Model file for the job. Use its own axes, mm. Face numbers are marked on the shaded views. Give positions to 0.01 mm unless a question says otherwise; leave off trailing zeros. Loops run counter-clockwise (first coordinate to the right, second up) from the corner with the lowest first, then second, coordinate; pieces in that order, holes last. Notation, with made-up numbers: M -16,-31.75 L 5,-31.75 A17 cw 5,-12.75 Z; hole C 86.5,42 d4. An arc over 180 degrees is marked long. Use CSV: the item, a comma, the result in double quotes. Start each with the question number.
(1) Slice it at B-B on z = 14. List the corners of the cut face in (x, y), and give its area (3 significant figures).
(2) Wall check: line 1 along X through (y, z) = (-7, 14); line 2 along Z through (x, y) = (-48, -2.25); line 3 along X through (y, z) = (-5, 4.5). Give the ranges that are in metal, low to high. Write a range as from..to.
(3) Flat gauge pins, fed straight in: P1, Ø3, axis at x = -18.21, z = 6, coming from the -Y side; P2, Ø10, axis at y = -11, z = 2.5, coming from the +X side; P3, Ø12, axis at y = -21.5, z = 15.5, coming from the +X side; P4, Ø2, axis at x = 23.5, z = 16.5, coming from the -Y side. Where does each tip first touch, or does it go through?
(4) Two-plate mould, pull along X, no slides. Class the marked faces 1, 2 and 3: pulls with the +X half, pulls with the -X half, needs draft (parallel to the pull), parting line crosses it, or undercut.
(5) Slice it at D-D on z = 3. List the corners of the cut face in (x, y), and give its area (3 significant figures).
(6) Slice it at A-A on x = 0. List the corners of the cut face in (y, z), and give its area (3 significant figures).
(7) Slice it at C-C on y = -15. List the corners of the cut face in (x, z).
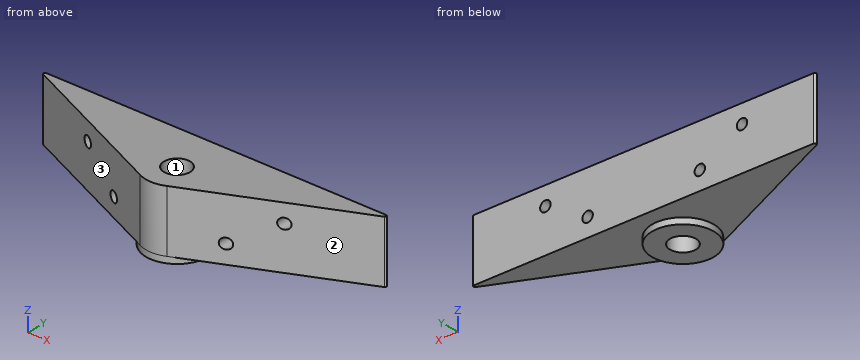
```python
from build123d import *

# Parameters (mm, degrees)
F0_R     = 4.2
F1_DEPTH = 20
F2_R     = 10
F2_R_2   = 4.2
F3_DEPTH = 2
F4_R     = 1.7
F5_DEPTH = 25


with BuildPart() as f1:
    # F0 (on Top) → F1 (new body)
    with BuildSketch(Plane.XY):
        with BuildLine():
            Line((-55.383945, -0.955682), (-4.349251, -24.004666))
            ThreePointArc((-4.349251, -24.004666), (0, -25), (4.349251, -24.004666))
            Line((4.349251, -24.004666), (55.383945, -0.955682))
            ThreePointArc((55.383945, -0.955682), (55.666938, -0.394741), (55.178144, 0))
            Line((55.178144, 0), (-55.178144, 0))
            ThreePointArc((-55.178144, 0), (-55.666938, -0.394741), (-55.383945, -0.955682))
        make_face()
        with Locations((0, -15)):
            Circle(F0_R, mode=Mode.SUBTRACT)
    extrude(amount=F1_DEPTH)

    # F2 (on face) → F3 (join)
    with BuildSketch(Plane(origin=(0, 0, 0), x_dir=(1, 0, 0), z_dir=(0, 0, -1))):
        with Locations((0, 15)):
            Circle(F2_R)
        with Locations((0, 15)):
            Circle(F2_R_2, mode=Mode.SUBTRACT)
    extrude(amount=F3_DEPTH)

    # F4 (on face) → F5 (cut)
    with BuildSketch(Plane(origin=(0, 0, 0), x_dir=(-1, 0, 0), z_dir=(0, 1, 0))):
        with Locations((-31.914174, 14)):
            Circle(F4_R)
        with Locations((-18.214174, 6)):
            Circle(F4_R)
        with Locations((18.214174, 6)):
            Circle(F4_R)
        with Locations((31.914174, 14)):
            Circle(F4_R)
    extrude(amount=-F5_DEPTH, mode=Mode.SUBTRACT)


solid = f1.part
```
Reply:
1,outline,"M -55.38,-0.96 L -33.61,-10.79 L -33.61,0 L -55.18,0 A0.5 ccw Z; M -30.21,-12.32 L -4.35,-24 A10 ccw 4.35,-24 L 30.21,-12.32 L 30.21,0 L -30.21,0 Z; M 33.61,-10.79 L 55.38,-0.96 A0.5 ccw 55.18,0 L 33.61,0 Z; hole C 0,-15 d8.4"
1,area,"1,350 mm^2"
2,line 1,"x = -42..-33.61, -30.21..30.21, 33.61..42"
2,line 2,"z = 0..20"
2,line 3,"x = -46.43..-19.01, -17.41..17.41, 19.01..46.43"
3,P1,"passes through"
3,P2,"stops at x = 44.21"
3,P3,"stops at x = 23.18"
3,P4,"stops at y = -15.81"
4,face 1,"undercut"
4,face 2,"pulls with the +X half"
4,face 3,"pulls with the -X half"
5,outline,"M -55.38,-0.96 L -4.35,-24 A10 ccw 4.35,-24 L 55.38,-0.96 A0.5 ccw 55.18,0 L -55.18,0 A0.5 ccw Z; hole C 0,-15 d8.4"
5,area,"1,430 mm^2"
6,outline,"M -25,-2 L -19.2,-2 L -19.2,20 L -25,20 Z; M -10.8,-2 L -5,-2 L -5,0 L 0,0 L 0,20 L -10.8,20 Z"
6,area,"355 mm^2"
7,outline,"M -24.29,0 L -10,0 L -10,-2 L -4.2,-2 L -4.2,20 L -24.29,20 Z; M 4.2,-2 L 10,-2 L 10,0 L 24.29,0 L 24.29,20 L 4.2,20 Z; hole C -18.21,6 d3.4; hole C 18.21,6 d3.4"
